Input: part model. Units: mm. Frame: model coordinates. A direction names the side the tool comes from. Give positions to 0.01 mm unless a question says otherwise; leave off trailing zeros. Order: outer loops, then holes, each group sorted by start corner. A loop starts at its lowest first (then second) coordinate and runs counter-clockwise, first axis right, second up. Notation, with made-up numbers: (63, 10.25) -> (83, 10.25) arc R22 cw to (83, 34.25) -> close; hole circle Ø6 at (55, -4.5). An arc over 180 degrees is marked (long way). Use a Markdown table: item, result. Add a question column.
Autodesk Inventor part; units mm, degrees
ref_plane "YZ Plane" through (0, 0, 0) normal (1, 0, 0) x (0, 1, 0)
ref_plane "XZ Plane" through (0, 0, 0) normal (0, 1, 0) x (-1, 0, 0)
ref_plane "XY Plane" through (0, 0, 0) normal (0, 0, 1) x (1, 0, 0)
sketch "Sketch1" plane through (0, 0, 0) normal (0, 1, 0) x (-1, 0, 0)
  line L0 (15, -15.715) -> (-15, -15.715)
  line L1 (-15, -15.715) -> (-15, 15.715)
  line L2 (-15, 15.715) -> (15, 15.715)
  line L3 (15, 15.715) -> (15, -15.715)
  point P0 (0, 0)
  dimension "d0" = 30
  dimension "d1" = 31.43
  dimension "d2" = 15
  dimension "d3" = 15.715
extrude "Plate1" add sketch "Sketch1" along normal blind 1.5
sketch "Sketch2" plane through (15, 0, 17.215) normal (0, 0, -1) x (-1, 0, 0)
  line L0 (30, 0) -> (0, 0)
  line L1 (0, 0) -> (0, 45)
  line L2 (0, 45) -> (30, 45)
  line L3 (30, 45) -> (30, 0)
edge flange "Flange1" height 45 angle 90 thickness 1.5 bend radius 0.31 thickness toward (0, 0, -1) relief tear relief width 1.5 relief depth 0.75 edges at (0, 1.5, 15.715) wall of the first edge with corners at (-15, 0, 17.215) (15, 0, 17.215) (15, 45, 17.215) (-15, 45, 17.215)
bend "Bend1"
corner "Corner1"
sketch "Sketch3" plane through (-15, 0, -17.215) normal (0, 0, 1) x (1, 0, 0)
  line L0 (30, 0) -> (0, 0)
  line L1 (0, 0) -> (0, 45)
  line L2 (0, 45) -> (30, 45)
  line L3 (30, 45) -> (30, 0)
edge flange "Flange2" height 45 angle 90 thickness 1.5 bend radius 0.31 thickness toward (0, 0, 1) relief tear relief width 1.5 relief depth 0.75 edges at (0, 1.5, -15.715) wall of the first edge with corners at (15, 0, -17.215) (-15, 0, -17.215) (-15, 45, -17.215) (15, 45, -17.215)
bend "Bend2"
corner "Corner2"
sketch "Sketch6" plane through (-15, 45, 17.215) normal (0, 0, 1) x (1, 0, 0)
  circle A0 centre (15, -10.5) radius 10
  line L0 (5, -10.5) -> (5, 9.5)
  line L1 (5, 9.5) -> (25, 9.5)
  line L2 (25, 9.5) -> (25, -10.5)
  line L3 (0, 0) -> (30, 0)
  line L4 (0, -43.19) -> (0, 0)
  line L5 (5.9376, -6.2723) -> (0, -19)
  line L6 (24.0624, -6.2723) -> (30, -19)
  line L7 (30, -45) -> (0, -45)
  line L8 (30, 0) -> (30, -43.19)
  point P0 (15, -45)
  point P1 (25, 0)
  point P2 (5, -8.2822)
  point P3 (5, 0)
  point P4 (30, -19)
  point P5 (25, -8.2822)
  dimension "d39" = 34.5
  dimension "d40" = 20
  dimension "d41" = 20
  dimension "d42" = 20
  dimension "d43" = 20
  dimension "d45" = 15
  dimension "d48" = 26
  dimension "d49" = 26
  dimension "d50" = 0
extrude "Extrusion1" cut sketch "Sketch6" against normal blind 50 contours A0 L5 L0 L3 L2 L6 | L2 L3 L8 L6 | L5 L4 L3 L0
sketch "Sketch7" plane through (-15, 1.81, 17.215) normal (0, 0, 1) x (1, 0, 0)
  arc A0 (24.0624, 36.9177) -> (5.9376, 36.9177) centre (15, 32.69) ccw
  circle A1 centre (22, 32.69) radius 1.05
  circle A2 centre (15, 39.69) radius 1.05
  circle A3 centre (8, 32.69) radius 1.05
  circle A4 centre (15, 25.69) radius 1.05
  point P0 (15, -1.81)
  dimension "d51" = 7
  dimension "d52" = 2.1
  dimension "d55" = 360
extrude "Extrusion2" cut sketch "Sketch7" against normal blind 20
sketch "Sketch8" plane through (0, 1.5, 0) normal (0, 1, 0) x (1, 0, 0)
  line L0 (15, 15.715) -> (9.0624, 15.715)
  line L1 (9.0624, 15.715) -> (-9.0624, 15.715)
  line L2 (-9.0624, 15.715) -> (-15, 15.715)
  line L3 (-15, 15.715) -> (15, 15.715)
  circle A0 centre (0, -2.285) radius 2.6
  point P0 (0, 0)
  point P1 (7, -2.285)
  point P2 (0, 4.715)
  point P3 (-7, -2.285)
  point P4 (0, -9.285)
  dimension "d59" = 18
  dimension "d60" = 0
  dimension "d61" = 5.2
  dimension "d62" = 7
  dimension "d63" = 0
  dimension "d66" = 360
extrude "Extrusion3" cut sketch "Sketch8" against normal blind 10
sketch "Sketch9" plane through (0, 1.5, 0) normal (0, 1, 0) x (1, 0, 0)
  point P0 (0, 0)
hole "Hole3" at (0, 1.5, -4.715) at (7, 1.5, 2.285) at (-7, 1.5, 2.285) at (0, 1.5, 9.285) direction (0, -1, 0) diameter 2.1 depth 1.5
hole "Hole4" at (0, 34.5, 17.215) direction (0, 0, -1) diameter 5.2 depth 1.5
sketch "Sketch10" plane through (15, 1.81, -17.215) normal (0, 0, -1) x (-1, 0, 0)
  circle A0 centre (15, 32.69) radius 2.6
  point P0 (15, -1.81)
hole "Hole5" at (0, 34.5, -17.215) direction (0, 0, 1) diameter 5.1 depth 1.5
equation "\"d75\" = Thickness"
equation "\"d82\" = Thickness"
equation "\"d89\" = Thickness"
equation "\"d4\" = Thickness"
equation "\"d5\" = BendReliefWidth"
equation "\"d6\" = BendReliefDepth"
equation "\"d7\" = MinimumRemnant"
equation "\"d8\" = TransitionRadius"
equation "\"d11\" = BendRadius"
equation "\"d12\" = CornerReliefSize"
equation "\"d13\" = GapSize"
equation "\"d14\" = JacobiRadiusSize"
equation "\"d15\" = BendReliefWidth"
equation "\"d16\" = BendReliefDepth"
equation "\"d17\" = MinimumRemnant"
equation "\"d18\" = TransitionRadius"
equation "\"d21\" = BendRadius"
equation "\"d22\" = CornerReliefSize"
equation "\"d23\" = GapSize"
equation "\"d24\" = JacobiRadiusSize"
equation "\"BendReliefWidth\" = Thickness"
equation "\"BendReliefDepth\" = 0.5 * Thickness"
equation "\"CornerReliefSize\" = 4 * Thickness"
equation "\"MinimumRemnant\" = 2 * Thickness"
equation "\"TransitionRadius\" = BendRadius"
equation "\"JacobiRadiusSize\" = BendRadius"
equation "\"GapSize\" = Thickness"
properties part number "axis_7_top_frame" material "Aluminum 6061-AHC"
Q1. Ray query, line 1 (X direction, y = 34, z = 16); line 2 (Z direction, x = 0, y = 0.35) (3 decimals); line 3 (Y direction, x = 9.5, z = 11). Return the intervals inside material, ascending.
Q2. Section query C-C (x = 0). Give the number of separate pieces and of enclosed holes in the cut face, plus the area to 3 significant figures.
Q3. Access query for faces 1 (the flat face through (4, 1.5, 0)), 2 (the flat face through (0, 19, -17.215)), 3 (the cylindrical face through (6.772, 33.475, 16.476)). Directions: +Z, -Z, +X, -X, +Y, -Y. A direction counts if a zero-diameter tool reaches every point of the face in a straight line with its end or side. Return the directions, or none.
Q4. Section query D-D (y = 34.5). Return loops of the section in (x, z) (3 decimals).
Q5. Draft query along Z for faces 4 (the cylindrical face through (-0.83, 40.86, 16.48)), 5 (the flat face through (0, 19, 17.215)), 6 (the cylindrical face through (-0.046, 0.74, 8.236)), 7 (the cylindrical face through (-7.315, 0.74, 3.287)). Return one class per face: +Z half, -Z half, draft (parallel to the pull), parting line (faces both ways), or undercut.
Q6. Section query B-B (y = 41.5). Return loops of the section in (x, z) (3 decimals).
Q7. Section query A-A (y = 8). Return loops of the section in (x, z) (3 decimals).
Q8. First-contact query: pin 1 (10 mm diameter, centred on y = 34, z = 11, fed in from -X); pin 2 (9 mm diameter, centred on x = 3, z = 4.5, fed in from +Y); pin 3 (1.9 mm diameter, centred on x = -7, y = 34.5, fed in from +Z) (3 decimals). Flat tips, straight axial feed; report the tip coordinate or a pass-through.
Solution:
| question | item | result |
|---|---|---|
| 1 | line 1 | x = -11.27 to -7.92, -6.08 to -2.55, 2.55 to 6.08, 7.92 to 11.27 |
| 1 | line 2 | z = -16.475 to -5.765, -3.665 to -0.315, 4.885 to 8.235, 10.335 to 16.475 |
| 1 | line 3 | y = 0 to 1.5 |
| 2 | separate pieces | 8 |
| 2 | enclosed holes | 0 |
| 2 | area | 143 mm² |
| 3 | face 1 | +X, -X, +Y |
| 3 | face 2 | -Z, +X, -X, +Y, -Y |
| 3 | face 3 | +Z |
| 4 | outline | (-11.035, -17.215) -> (-2.55, -17.215) -> (-2.55, -15.715) -> (-11.035, -15.715) -> close; (-11.035, 15.715) -> (-8.05, 15.715) -> (-8.05, 17.215) -> (-11.035, 17.215) -> close; (-5.95, 15.715) -> (-2.6, 15.715) -> (-2.6, 17.215) -> (-5.95, 17.215) -> close; (2.55, -17.215) -> (11.035, -17.215) -> (11.035, -15.715) -> (2.55, -15.715) -> close; (2.6, 15.715) -> (5.95, 15.715) -> (5.95, 17.215) -> (2.6, 17.215) -> close; (8.05, 15.715) -> (11.035, 15.715) -> (11.035, 17.215) -> (8.05, 17.215) -> close |
| 5 | face 4 | draft |
| 5 | face 5 | +Z half |
| 5 | face 6 | undercut |
| 5 | face 7 | undercut |
| 6 | outline | (-7.141, -17.215) -> (7.141, -17.215) -> (7.141, -15.715) -> (-7.141, -15.715) -> close; (-7.141, 15.715) -> (-1.05, 15.715) -> (-1.05, 17.215) -> (-7.141, 17.215) -> close; (1.05, 15.715) -> (7.141, 15.715) -> (7.141, 17.215) -> (1.05, 17.215) -> close |
| 7 | outline | (-15, -17.215) -> (15, -17.215) -> (15, -15.715) -> (-15, -15.715) -> close; (-15, 15.715) -> (15, 15.715) -> (15, 17.215) -> (-15, 17.215) -> close |
| 8 | pin 1 | stops at x = -12.04 |
| 8 | pin 2 | stops at y = 1.5 |
| 8 | pin 3 | stops at z = -15.715 |
